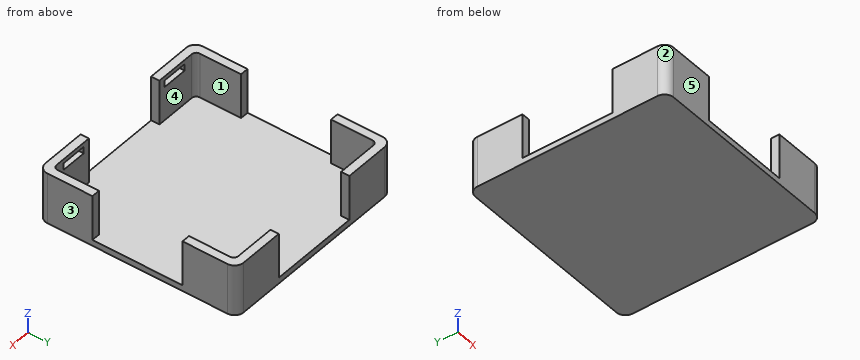
from build123d import *

# Parameters (mm, degrees)
PAD001_DEPTH = 2
PAD002_DEPTH = 15
SKETCH003_W  = 2.25
SKETCH003_H  = 8.5
POCKET_DEPTH = 2


with BuildPart() as part:
    # Sketch001 → Pad001 (new body)
    with BuildSketch(Plane.XY):
        with BuildLine():
            Line((-30, 33), (30, 33))
            ThreePointArc((33, 30), (32.12132, 32.12132), (30, 33))
            Line((33, 30), (33, -30))
            ThreePointArc((30, -33), (32.12132, -32.12132), (33, -30))
            Line((30, -33), (-30, -33))
            ThreePointArc((-33, -30), (-32.12132, -32.12132), (-30, -33))
            Line((-33, -30), (-33, 30))
            ThreePointArc((-30, 33), (-32.12132, 32.12132), (-33, 30))
        make_face()
    extrude(amount=PAD001_DEPTH)

    # Sketch002 (on Face10 of Pad001) → Pad002 (join)
    with BuildSketch(Plane.XY.offset(2)):
        with BuildLine():
            ThreePointArc((-30, 33), (-32.12132, 32.12132), (-33, 30))
            Line((-33, 30), (-33, 15))
            Line((-33, 15), (-30.25, 15))
            Line((-30.25, 15), (-30.25, 28.75))
            ThreePointArc((-28.75, 30.25), (-29.81066, 29.81066), (-30.25, 28.75))
            Line((-15, 30.25), (-28.75, 30.25))
            Line((-15, 33), (-15, 30.25))
            Line((-30, 33), (-15, 33))
        make_face()
        with BuildLine():
            ThreePointArc((33, 30), (32.12132, 32.12132), (30, 33))
            Line((30, 33), (15, 33))
            Line((15, 33), (15, 30.25))
            Line((15, 30.25), (28.75, 30.25))
            ThreePointArc((30.25, 28.75), (29.81066, 29.81066), (28.75, 30.25))
            Line((30.25, 15), (30.25, 28.75))
            Line((33, 15), (30.25, 15))
            Line((33, 30), (33, 15))
        make_face()
        with BuildLine():
            ThreePointArc((-33, -30), (-32.12132, -32.12132), (-30, -33))
            Line((-30, -33), (-15, -33))
            Line((-15, -33), (-15, -30.25))
            Line((-15, -30.25), (-28.75, -30.25))
            ThreePointArc((-30.25, -28.75), (-29.81066, -29.81066), (-28.75, -30.25))
            Line((-30.25, -15), (-30.25, -28.75))
            Line((-33, -15), (-30.25, -15))
            Line((-33, -30), (-33, -15))
        make_face()
        with BuildLine():
            ThreePointArc((30, -33), (32.12132, -32.12132), (33, -30))
            Line((33, -30), (33, -15))
            Line((33, -15), (30.25, -15))
            Line((30.25, -15), (30.25, -28.75))
            ThreePointArc((28.75, -30.25), (29.81066, -29.81066), (30.25, -28.75))
            Line((15, -30.25), (28.75, -30.25))
            Line((15, -33), (15, -30.25))
            Line((30, -33), (15, -33))
        make_face()
    extrude(amount=PAD002_DEPTH)

    # Sketch003 (on DatumPlane) → Pocket (cut)
    with BuildSketch(Plane(origin=(0, -30.25, 9.5), x_dir=(0, 0, 1), z_dir=(0, 1, 0))):
        with Locations((4.975, -21.5)):
            Rectangle(SKETCH003_W, SKETCH003_H)
        with Locations((4.975, 21.5)):
            Rectangle(SKETCH003_W, SKETCH003_H)
    extrude(amount=-POCKET_DEPTH, mode=Mode.SUBTRACT)


with BuildPart() as part_1:
    # Body001 placement: moved
    add(part.part.moved(Location((0, 0, -17))))


solid = part_1.part
Source: CAD feature listing. Evaluate the final solid. Frame: model axes, mm. Face numbers are marked on the shaded views. A direction names the side the tool comes from. Round coordinates to 2 decimals unless told otherwise and drop trailing zeros. Loops run counter-clockwise (first coordinate to the right, second up) from the corner with the lowest first, then second, coordinate; pieces in that order, holes last.
Q1. Ray query, line 1 (Y direction, x = -28.5, z = -3); line 2 (Z direction, x = -24, y = 12.5). Return the intervals inside material, ascending.
Q2. First-contact query: P1, Ø1, axis at y = -31, z = -2.5, coming from the -X side; P2, Ø3, axis at x = 22, y = 17, coming from the +Z side; P3, Ø1, axis at y = -31.5, z = -2, coming from the +X side. Flat tips, straight axial feed; report the tip coordinate or a pass-through.
Q3. Section D-D, the plane x = -16. Return loops of the section in (y, z), plus the area to 4 significant figures.
Q4. Access query for the marked faces 1 and 2. Directions: +Z, -Z, +X, -X, +Y, -Y. A direction counts if a zero-diameter tool reaches every point of the face in a straight line with its end or side. Return the directions, or none.
Q5. Mould query, pull axis X, two halves, no side actions, for the marked faces 3, 4 and 5. Classes: pulls with the +X half, pulls with the -X half, needs draft (parallel to the pull), parting line crosses it, or undercut.
Q6. Section B-B, the plane x = -24. Return loops of the section in (y, z), plus the area to 3 significant figures.
Q7. Section A-A, the plane z = -11.5. State how many separate pieces and enclosed holes the cut face has, plus the area to 3 significant figures.
Q8. Section C-C, the plane y = 5. Return loops of the section in (x, z), plus the area to 3 significant figures.
Solutions:
1. line 1: y = -33 to -30.25, 30.25 to 33
1. line 2: z = -17 to -15
2. P1: stops at x = -32.96
2. P2: stops at z = -15
2. P3: stops at x = 32.83
3. outline: (-33, -17) - (33, -17) - (33, 0) - (30.25, 0) - (30.25, -15) - (-30.25, -15) - (-30.25, 0) - (-33, 0) - close
3. area: 214.5 mm2
4. face 1: +Z
4. face 2: +Z, -Z, -X, -Y
5. face 3: pulls with the +X half
5. face 4: undercut
5. face 5: needs draft
6. outline: (-33, -17) - (33, -17) - (33, 0) - (30.25, 0) - (30.25, -15) - (-30.25, -15) - (-30.25, -3.65) - (-32.25, -3.65) - (-32.25, -1.4) - (-30.25, -1.4) - (-30.25, 0) - (-33, 0) - close
6. area: 210 mm2
7. separate pieces: 4
7. enclosed holes: 0
7. area: 360 mm2
8. outline: (-33, -17) - (33, -17) - (33, -15) - (-33, -15) - close
8. area: 132 mm2
